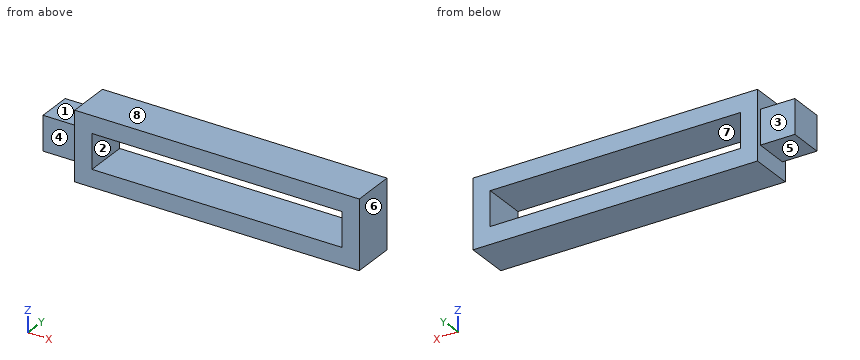
from build123d import *

# Parameters (mm, degrees)
SKETCH1_W                = 660
SKETCH1_H                = 160
SKETCH1_W_2              = 580
SKETCH1_H_2              = 80
BOSS_EXTRUDE1_DEPTH      = 50
BOSS_EXTRUDE1_DEPTH_BACK = 50
SKETCH1_3_W              = 80
SKETCH1_3_H              = 80
BOSS_EXTRUDE2_DEPTH      = 40
BOSS_EXTRUDE2_DEPTH_BACK = 40


with BuildPart() as part:
    # Sketch1 → Boss-Extrude1 (new body, two sides)
    with BuildSketch(Plane(origin=(0, 0, 0), x_dir=(1, 0, 0), z_dir=(0, 1, 0))) as boss_extrude1_sk:
        Rectangle(SKETCH1_W, SKETCH1_H)
        Rectangle(SKETCH1_W_2, SKETCH1_H_2, mode=Mode.SUBTRACT)
    extrude(amount=BOSS_EXTRUDE1_DEPTH)
    extrude(boss_extrude1_sk.sketch, amount=-BOSS_EXTRUDE1_DEPTH_BACK)

    # Sketch1_3 → Boss-Extrude2 (add, two sides)
    with BuildSketch(Plane(origin=(0, 0, 0), x_dir=(1, 0, 0), z_dir=(0, 1, 0))) as boss_extrude2_sk:
        with Locations((-370, 0)):
            Rectangle(SKETCH1_3_W, SKETCH1_3_H)
    extrude(amount=BOSS_EXTRUDE2_DEPTH)
    extrude(boss_extrude2_sk.sketch, amount=-BOSS_EXTRUDE2_DEPTH_BACK)


solid = part.part
Geometry check sheet. Reference: the model listing, model coordinates, mm. Face numbers are marked on the shaded views. A direction names the side the tool comes from. Give positions to 0.01 mm unless a question says otherwise; leave off trailing zeros. Write each loop counter-clockwise with the first axis right and the second up, starting at its lowest first coordinate (ties: lowest second). Pieces come first, ordered by that corner, then holes. Notation, with made-up numbers: (20.5, -12) - (63.5, -12) arc R27 ccw to (63.5, 14) - close; hole circle Ø3 at (67.25, 6.5). An arc over 180 degrees is marked (long way). Put each result on its own line as item: value.
1. Sectioned sample at C-C, the plane y = 5. Enter the section's corners in (x, z).
Ans:
outline: (-410, -40) - (-330, -40) - (-330, -80) - (330, -80) - (330, 80) - (-330, 80) - (-330, 40) - (-410, 40) - close; hole (-290, -40) - (290, -40) - (290, 40) - (-290, 40) - close
2. Sectioned sample at B-B, the plane z = -10.5. Enter the section's corners in (x, y), plus the area to 3 significant figures.
Ans:
outline: (-410, -40) - (-330, -40) - (-330, -50) - (-290, -50) - (-290, 50) - (-330, 50) - (-330, 40) - (-410, 40) - close; (290, -50) - (330, -50) - (330, 50) - (290, 50) - close
area: 14,400 mm²
3. Set-up check for the marked faces 4, 5, 6, 7 and 8: record each of +Z, -Z, +X, -X, +Y, -Y from which the full face is reachable in a straight line by a thin tool's end or side.
Ans:
face 4: +Z, -Z, -X, -Y
face 5: -Z, -X, +Y, -Y
face 6: +Z, -Z, +X, +Y, -Y
face 7: +Y, -Y
face 8: +Z, +X, -X, +Y, -Y
4. Sectioned sample at D-D, the plane z = -53. Enter the section's corners in (x, y), plus the area to 3 significant figures.
Ans:
outline: (-330, -50) - (330, -50) - (330, 50) - (-330, 50) - close
area: 66,000 mm²
5. Draft check along Z on the marked faces 1, 2 and 3. Enter one of: +Z half, -Z half, draft (parallel to the pull), parting line (faces both ways), or undercut.
Ans:
face 1: +Z half
face 2: undercut
face 3: draft
6. Go/stop test with a flat-tipped pin: pin 1 (24 mm diameter, centred on x = -375.5, z = -16, fed in from -Y). Record where the tip stops, or that it passes through.
Ans:
pin 1: stops at y = -40
7. Sectioned sample at A-A, the plane x = 199.5. Enter the section's corners in (y, z), plus the area to 3 significant figures.
Ans:
outline: (-50, -80) - (50, -80) - (50, -40) - (-50, -40) - close; (-50, 40) - (50, 40) - (50, 80) - (-50, 80) - close
area: 8,000 mm²
8. Thickness scan on line 1 (X direction, y = 35, z = -35.5); line 2 (Z direction, x = -160, y = 3); line 3 (X direction, y = 40.5, z = -31). Record the ranges inside material, lowest first.
Ans:
line 1: x = -410 to -290, 290 to 330
line 2: z = -80 to -40, 40 to 80
line 3: x = -330 to -290, 290 to 330
